Geometry check sheet. Reference: the model listing, model coordinates, mm. A direction names the side the tool comes from. Coordinates: 2 decimals unless noted, no trailing zeros. Order: outer loops, then holes, each group sorted by start corner. A loop starts at its lowest first (then second) coordinate and runs counter-clockwise, first axis right, second up. Notation, with made-up numbers: (-24.75, 31) - (-19.75, 31) arc R15 cw to (-19.75, 41) - close; hole circle Ø7 at (59.25, 45.5). An arc over 180 degrees is marked (long way). Return JSON: item names as keys, results as strings. Group by question number.
Item 1: Gauge pin test, flat ends, axial feed: pin 1 (5 mm diameter, centred on y = -51.5, z = 6, fed in from -X); pin 2 (1.5 mm diameter, centred on x = 93, z = 8, fed in from +Y); pin 3 (0.8 mm diameter, centred on x = 62, y = -94.5, fed in from +Z); pin 4 (2 mm diameter, centred on x = 87, y = -13.5, fed in from -Z). Record the tip position at first contact, or that the pin passes through.
Item 2: Section check A-A on y = -53.5. Enter the section's corners in (x, z), then the cut area to 3 significant figures.
Item 3: Tool access check on faces 4 (the flat face through (111, -53, 5)), 5 (the flat face through (0, 3, 7)). Record the directions out of +Z, -Z, +X, -X, +Y, -Y that give a thin tool (end or side, any length) a straight path to the whole face; none if there is none.
Item 4: Section check C-C on x = 103. Enter the section's corners in (y, z), then the cut area to 3 significant figures.
Item 5: Scan lines: probe 1 along Z at (x, y) = (114, -4.5); probe 2 along Y at (x, z) = (77, 4); probe 3 along Y at (x, z) = (83.5, 9.75). Record each from-to range of solid material in increasing order.
Item 6: Section check B-B on x = 86.5. Enter the section's corners in (y, z).
Item 7: Draft check along X on faces 1 (the flat face through (2.5, -50, 3)), 2 (the cylindrical face through (48.94, -98.53, 1.23)), 3 (the flat face through (65.2, -50, 3)). Enter one of: pulls with the +X half, pulls with the -X half, needs draft (parallel to the pull), parting line crosses it, or undercut.
Item 8: Section check D-D on z = 2.25. Enter the section's corners in (x, y).
from build123d import *

# Parameters (mm, degrees)
BOSS_EXTRUDE1_DEPTH = 5
BOSS_EXTRUDE2_DEPTH = 20
CUT_EXTRUDE1_DEPTH  = 157.917080014
FILLET1_R           = 5
CUT_EXTRUDE6_DEPTH  = 159.804030176
SKETCH5_R           = 6
CUT_EXTRUDE7_DEPTH  = 3.5
FILLET2_R           = 5
SKETCH6_W           = 115.4
SKETCH6_H           = 1
BOSS_EXTRUDE3_DEPTH = 0.5


with BuildPart() as part:
    # Sketch1 → Boss-Extrude1 (new body)
    with BuildSketch(Plane.XY):
        Polygon((25.2, 0), (25.2, -101.6), (37.9, -101.6), (37.9, 0), (42.5, 0), (42.5, -101.6), (55.2, -101.6), (55.2, 0), (65.2, 0), (65.2, -101.6), (77.9, -101.6), (77.9, 0), (82.5, 0), (82.5, -101.6), (95.2, -101.6), (95.2, 0), (105.2, 0), (105.2, -101.6), (117.9, -101.6), (117.9, 0), (120.4, 0), (120.4, 6), (0, 6), (0, 0), (2.5, 0), (2.5, -101.6), (15.2, -101.6), (15.2, 0), align=None)
    extrude(amount=BOSS_EXTRUDE1_DEPTH)

    # Sketch1<3> → Boss-Extrude2 (add)
    with BuildSketch(Plane.XY):
        Polygon((15.2, 0), (25.2, 0), (37.9, 0), (42.5, 0), (55.2, 0), (65.2, 0), (77.9, 0), (82.5, 0), (95.2, 0), (105.2, 0), (117.9, 0), (120.4, 0), (120.4, 6), (0, 6), (0, 0), (2.5, 0), align=None)
    extrude(amount=BOSS_EXTRUDE2_DEPTH)

    # Sketch2 → Cut-Extrude1 (cut, through all)
    with BuildSketch(Plane(origin=(117.9, 0, 0), x_dir=(0, 0, -1), z_dir=(1, 0, 0))):
        with BuildLine():
            Line((-3.771412758, -101.6), (0, -101.6))
            Line((0, -101.6), (0, -94.860498406))
            ThreePointArc((0, -94.860498406), (-1.259194033, -98.580844365), (-3.771412758, -101.6))
        make_face()
    extrude(amount=-CUT_EXTRUDE1_DEPTH, mode=Mode.SUBTRACT)

    # Fillet1
    fillet1_edges = [part.edges().sort_by_distance(p)[0] for p in [
        (8.85, 0, 5),
        (31.55, 0, 5),
        (48.85, 0, 5),
        (71.55, 0, 5),
        (88.85, 0, 5),
        (111.55, 0, 5),
    ]]
    fillet(fillet1_edges, radius=FILLET1_R)

    # Sketch4 → Cut-Extrude6 (cut, through all)
    with BuildSketch(Plane(origin=(120.4, 0, 0), x_dir=(0, 0, -1), z_dir=(1, 0, 0))):
        Polygon((0, 6), (-20, 4.250226729), (-20, 6), align=None)
    extrude(amount=-CUT_EXTRUDE6_DEPTH, mode=Mode.SUBTRACT)

    # Sketch5 → Cut-Extrude7 (cut)
    with BuildSketch(Plane(origin=(0, 5.954423259, 0.520944533), x_dir=(1, 0, 0), z_dir=(0, 0.9961946980917462, 0.08715574274765159))):
        with Locations(Location((110.4, -9.553462294, 0), (0, 0, 270))):
            Circle(SKETCH5_R)
        with Locations(Location((10, -9.553462294, 0), (0, 0, 270))):
            Circle(SKETCH5_R)
    extrude(amount=-CUT_EXTRUDE7_DEPTH, mode=Mode.SUBTRACT)

    # Fillet2
    fillet2_edges = [part.edges().sort_by_distance(p)[0] for p in [
        (0, 2.125113365, 20),
        (120.4, 2.125113365, 20),
    ]]
    fillet(fillet2_edges, radius=FILLET2_R)

    # Sketch6 → Boss-Extrude3 (add)
    with BuildSketch(Plane.XY):
        with Locations((60.2, -94.360498406)):
            Rectangle(SKETCH6_W, SKETCH6_H)
    extrude(amount=BOSS_EXTRUDE3_DEPTH)


solid = part.part
Computed:
{
 "1": {"pin 1": "stops at x = 2.5", "pin 2": "stops at y = 5.37", "pin 3": "stops at z = 0.5", "pin 4": "stops at z = 0"},
 "2": {"outline": "(2.5, 0) - (15.2, 0) - (15.2, 5) - (2.5, 5) - close; (25.2, 0) - (37.9, 0) - (37.9, 5) - (25.2, 5) - close; (42.5, 0) - (55.2, 0) - (55.2, 5) - (42.5, 5) - close; (65.2, 0) - (77.9, 0) - (77.9, 5) - (65.2, 5) - close; (82.5, 0) - (95.2, 0) - (95.2, 5) - (82.5, 5) - close; (105.2, 0) - (117.9, 0) - (117.9, 5) - (105.2, 5) - close", "area": "381 mm²"},
 "3": {"face 4": "+Z, +X, -X, -Y", "face 5": "+Z, -Z, -X, +Y, -Y"},
 "4": {"outline": "(-94.86, 0) - (-93.86, 0) - (-93.86, 0.5) - (-94.86, 0.5) - close; (0, 0) - (6, 0) - (4.25, 20) - (0, 20) - close", "area": "103 mm²"},
 "5": {"probe 1": "z = 0 to 5.03", "probe 2": "y = -101.6 to 5.65", "probe 3": "y = -0.01 to 5.15"},
 "6": {"outline": "(-101.6, 3.77) arc R10.74 ccw to (-94.86, 0) - (6, 0) - (4.25, 20) - (0, 20) - (0, 10) arc R5 cw to (-5, 5) - (-101.6, 5) - close"},
 "7": {"face 1": "pulls with the -X half", "face 2": "needs draft", "face 3": "undercut"},
 "8": {"outline": "(0, 0) - (2.5, 0) - (2.5, -100.05) - (15.2, -100.05) - (15.2, 0) - (25.2, 0) - (25.2, -100.05) - (37.9, -100.05) - (37.9, 0) - (42.5, 0) - (42.5, -100.05) - (55.2, -100.05) - (55.2, 0) - (65.2, 0) - (65.2, -100.05) - (77.9, -100.05) - (77.9, 0) - (82.5, 0) - (82.5, -100.05) - (95.2, -100.05) - (95.2, 0) - (105.2, 0) - (105.2, -100.05) - (117.9, -100.05) - (117.9, 0) - (120.4, 0) - (120.4, 5.8) - (0, 5.8) - close"}
}
